Part model, mm, in its own coordinate system. A direction names the side the tool comes from. Round coordinates to 2 decimals unless told otherwise and drop trailing zeros. Write each loop counter-clockwise with the first axis right and the second up, starting at its lowest first coordinate (ties: lowest second). Pieces come first, ordered by that corner, then holes. Notation, with made-up numbers: (32, 88) -> (89, 88) arc R19 cw to (89, 121) -> close; hole circle Ø6 at (62, -16). An arc over 180 degrees is marked (long way). Return JSON: item names as keys, results as strings. Group by question number.
(1) Tool access for faces 4 (the cylindrical face through (19.01, -49.19, 16.95)), 5 (the flat face through (15, -76.2, 25)): list every direction of +Z, -Z, +X, -X, +Y, -Y with a clear straight run to the whole face (end or side of a thin tool).
(2) Saw through at C-C (y = 9.5). List the corners of the cut face in (x, z) (1 decimal).
(3) Saw through at B-B (x = 25.4). List the corners of the cut face in (y, z), plus the area to 3 significant figures.
(4) Saw through at D-D (x = 32). List the corners of the cut face in (y, z).
(5) Saw through at A-A (z = 25.4). List the corners of the cut face in (x, y).
(6) Drop flat-ended pins along their axis: pin 1 Ø4 at (y, z) = (-54, 13) entering from +X; pin 2 Ø12 at (x, z) = (10, 39.5) entering from -Y; pin 3 Ø10 at (x, y) = (17.5, -55.5) entering from +Z (3 decimals); pin 4 Ø1 at (x, z) = (27, 17.5) entering from +Y. Give the stop position or say it passes through.
(7) Drill centre lines: L1, parallel to Y at x = 11, z = 36.5; L2, parallel to Y at x = 12, z = 21; L3, parallel to X at y = 2, z = 23. Where is each one in solid material? Low to high. Write a range as from..to.
(8) Mould opens along X. For faces 1 (the flat face through (23, -25.4, 20)), 2 (the cylindrical face through (27.96, 12.522, 29.416)), 3 (the flat face through (0, -13, 25)) say: +X half, -X half, draft (parallel to the pull), parting line (faces both ways), or undercut.
from build123d import *

# Parameters (mm, degrees)
F0_W     = 38.1
F0_H     = 50.8
F1_DEPTH = 25.4
F2_R     = 9.525
F3_DEPTH = 50.8
F4_R     = 2.54
F6_R     = 4.7625
F7_DEPTH = 25.4


with BuildPart() as f1:
    # F0 (on Front) → F1 (new body)
    with BuildSketch(Plane.XZ):
        with Locations((19.05, 25.4)):
            Rectangle(F0_W, F0_H)
    extrude(amount=F1_DEPTH)

    # F2 (on face) → F3 (join)
    with BuildSketch(Plane.XZ.offset(25.4)):
        with Locations((14.613638, 25.4)):
            Circle(F2_R)
    extrude(amount=F3_DEPTH)

    # F4
    f4_edges = [f1.edges().sort_by_distance(p)[0] for p in [
        (5.088638, -76.2, 25.4),
    ]]
    fillet(f4_edges, radius=F4_R)

    # F6 (on face) → F7 (join)
    with BuildSketch(Plane.XZ):
        with Locations((25.4, 25.4)):
            Circle(F6_R)
    extrude(amount=-F7_DEPTH)


solid = f1.part
Computed values:
{
 "1": {"face 4": "-Y", "face 5": "+Z, -Z, +X, -X, -Y"},
 "2": {"outline": "circle Ø9.5 at (25.4, 25.4)"},
 "3": {"outline": "(-25.4, 0) -> (0, 0) -> (0, 20.64) -> (25.4, 20.64) -> (25.4, 30.16) -> (0, 30.16) -> (0, 50.8) -> (-25.4, 50.8) -> close", "area": "1,530 mm2"},
 "4": {"outline": "(-25.4, 0) -> (0, 0) -> (0, 50.8) -> (-25.4, 50.8) -> close"},
 "5": {"outline": "(0, -25.4) -> (5.09, -25.4) -> (5.09, -73.66) arc R2.54 ccw to (7.63, -76.2) -> (21.6, -76.2) arc R2.54 ccw to (24.14, -73.66) -> (24.14, -25.4) -> (38.1, -25.4) -> (38.1, 0) -> (30.16, 0) -> (30.16, 25.4) -> (20.64, 25.4) -> (20.64, 0) -> (0, 0) -> close"},
 "6": {"pin 1": "through", "pin 2": "y = -75.4", "pin 3": "z = 34.925", "pin 4": "y = 0"},
 "7": {"L1": "-25.4..0", "L2": "-76.2..0", "L3": "21.29..29.51"},
 "8": {"face 1": "draft", "face 2": "parting line", "face 3": "-X half"}
}
